Verification items for the finished model (mm, model axes). Give positions to 0.01 mm unless a question says otherwise; leave off trailing zeros. Order: outer loops, then holes, each group sorted by start corner. A loop starts at its lowest first (then second) coordinate and runs counter-clockwise, first axis right, second up.
(1) Gauge pin test, flat end, axial feed: pin 1 (1.8 mm diameter, centred on x = -8.5, y = 0, fed in from -Z). Record the tip position at first contact, or that the pin passes through.
(2) Mould release check, pull along Y, two halves, no side actions. Record for faces 1 (the face through (15.14, 15.1, 1.48)), 2 (the face through (16, 0, 1)), 3 (the face through (-10, 0, 2)): pulls with the +Y half, pulls with the -Y half, needs draft (parallel to the pull), parting line crosses it, or undercut.
(3) Sectioned sample at D-D on y = -12. Record the cut outline in (x, z).
(4) Scan lines: L1, parallel to Y at x = 8.5, z = 2; L2, parallel to Y at x = -13.5, z = 1.25; L3, parallel to Y at x = 5.5, z = 1.2. Record each from-to range of solid material in increasing order.
(5) Sectioned sample at C-C on z = 0.8. Count the separate pieces of the cut face and the enclosed holes in it, plus the area to 3 significant figures.
(6) Sectioned sample at B-B on y = 0. Record the cut outline in (x, z).
(7) Sectioned sample at A-A on x = 0. Record the cut outline in (y, z), plus the area to 3 significant figures.
```python
from build123d import *

# Parameters (mm, degrees)
BOSS_EXTRU_1_DEPTH      = 3
ESQUISSE2_R             = 6
ESQUISSE2_R_2           = 1.5
ENL_V_MAT_EXTRU_1_DEPTH = 23.825424421
ESQUISSE3_R             = 1.5
ENL_V_MAT_EXTRU_2_DEPTH = 23.825424421


with BuildPart() as part:
    # Esquisse1 → Boss.-Extru.1 (new body)
    with BuildSketch(Plane.XY):
        with BuildLine():
            Line((-13, -16), (13, -16))
            ThreePointArc((13, -16), (15.121320344, -15.121320344), (16, -13))
            Line((16, -13), (16, 13))
            ThreePointArc((16, 13), (15.121320344, 15.121320344), (13, 16))
            Line((13, 16), (-13, 16))
            ThreePointArc((-13, 16), (-15.121320344, 15.121320344), (-16, 13))
            Line((-16, 13), (-16, -13))
            ThreePointArc((-16, -13), (-15.121320344, -15.121320344), (-13, -16))
        make_face()
    extrude(amount=BOSS_EXTRU_1_DEPTH)

    # Esquisse2 → Enlèv. mat.-Extru.1 (cut, through all)
    with BuildSketch(Plane.XY.offset(3)):
        Circle(ESQUISSE2_R)
        with Locations((-8.5, 0)):
            Circle(ESQUISSE2_R_2)
        with Locations((-6.01040764, 6.01040764)):
            Circle(ESQUISSE2_R_2)
        with Locations(Location((-6.01040764, -6.01040764, 0), (0, 0, 180))):
            Circle(ESQUISSE2_R_2)
        with Locations((6.01040764, -6.01040764)):
            Circle(ESQUISSE2_R_2)
        with Locations(Location((8.5, 0, 0), (0, 0, 180))):
            Circle(ESQUISSE2_R_2)
        with Locations(Location((6.01040764, 6.01040764, 0), (0, 0, 180))):
            Circle(ESQUISSE2_R_2)
    extrude(amount=-ENL_V_MAT_EXTRU_1_DEPTH, mode=Mode.SUBTRACT)

    # Esquisse3 → Enlèv. mat.-Extru.2 (cut, through all)
    with BuildSketch(Plane.XY.offset(3)):
        with Locations((-13, 13)):
            Circle(ESQUISSE3_R)
        with Locations(Location((13, 13, 0), (0, 0, 180))):
            Circle(ESQUISSE3_R)
        with Locations((13, -13)):
            Circle(ESQUISSE3_R)
        with Locations(Location((-13, -13, 0), (0, 0, 180))):
            Circle(ESQUISSE3_R)
    extrude(amount=-ENL_V_MAT_EXTRU_2_DEPTH, mode=Mode.SUBTRACT)


solid = part.part
```
Ans:
1. pin 1: passes through
2. face 1: pulls with the +Y half
2. face 2: needs draft
2. face 3: undercut
3. outline: (-16, 0) - (-14.12, 0) - (-14.12, 3) - (-16, 3) - close; (-11.88, 0) - (11.88, 0) - (11.88, 3) - (-11.88, 3) - close; (14.12, 0) - (16, 0) - (16, 3) - (14.12, 3) - close
4. L1: y = -16 to -1.5, 1.5 to 16
4. L2: y = -15.96 to -14.41, -11.59 to 11.59, 14.41 to 15.96
4. L3: y = -16 to -7.42, -4.6 to -2.4, 2.4 to 4.6, 7.42 to 16
5. separate pieces: 1
5. enclosed holes: 11
5. area: 832 mm2
6. outline: (-16, 0) - (-10, 0) - (-10, 3) - (-16, 3) - close; (-7, 0) - (-6, 0) - (-6, 3) - (-7, 3) - close; (6, 0) - (7, 0) - (7, 3) - (6, 3) - close; (10, 0) - (16, 0) - (16, 3) - (10, 3) - close
7. outline: (-16, 0) - (-6, 0) - (-6, 3) - (-16, 3) - close; (6, 0) - (16, 0) - (16, 3) - (6, 3) - close
7. area: 60.0 mm2
